Read the model definition and answer for the solid it produces. Units are mm, in the model's axes. Face numbers are marked on the shaded views. Give positions to 0.01 mm unless a question says otherwise; leave off trailing zeros. Write each loop counter-clockwise with the first axis right and the second up, starting at its lowest first coordinate (ties: lowest second). Pieces come first, ordered by that corner, then holes. Notation, with made-up numbers: (84.25, 69.5) - (88.25, 69.5) arc R13 ccw to (88.25, 83.5) - close; hole circle Ø9 at (-32, -11). An arc over 180 degrees is marked (long way). Answer as a JSON object with one key per item and string values. Group by question number.
```python
from build123d import *

# Parameters (mm, degrees)
F0_W     = 220
F0_H     = 50
F0_R     = 17.5
F0_R_2   = 7.5
F1_DEPTH = 20
F2_D     = 13.2
F3_R     = 5


with BuildPart() as f1:
    # F0 (on Top) → F1 (new body)
    with BuildSketch(Plane.XY):
        Rectangle(F0_W, F0_H)
        with Locations((-50, 0)):
            Circle(F0_R, mode=Mode.SUBTRACT)
        Circle(F0_R_2, mode=Mode.SUBTRACT)
        with Locations((50, 0)):
            Circle(F0_R, mode=Mode.SUBTRACT)
    extrude(amount=F1_DEPTH)

    # F2 (through all)
    with Locations(Plane(origin=(0, 0, 0), x_dir=(1, 0, 0), z_dir=(0, 0, -1))):
        with Locations((-95, -12.5), (-95, 12.5), (95, -12.5), (95, 12.5)):
            Hole(F2_D / 2)

    # F3
    f3_edges = [f1.edges().sort_by_distance(p)[0] for p in [
        (-110, -25, 10),
        (110, -25, 10),
        (110, 25, 10),
        (-110, 25, 10),
    ]]
    fillet(f3_edges, radius=F3_R)


solid = f1.part
```
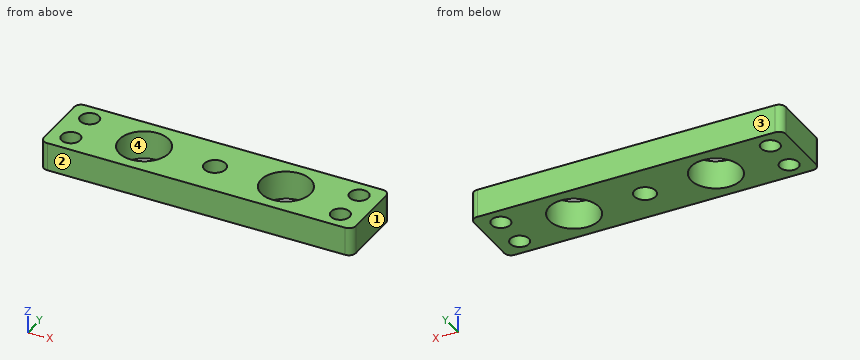
1) Find section D-D, the plane y = -12.5. Write down the section's boundary in (x, z), and give its area (3 significant figures).
2) Find section B-B, the plane y = 0. Write down the section's boundary in (x, z), and give its area (3 significant figures).
3) Find section C-C, the plane x = 0. Write down the section's boundary in (y, z), and give its area (3 significant figures).
4) Find the intervals of material crossed by line 1 (Y direction, x = -95, z = 12.25); line 2 (Y direction, x = -50, z = 8.25); line 3 (X direction, y = 2.5, z = 17.75), in increasing order. Write a range as [from, to].
5) For a pull along Y with two mould halves and no side action, classify the marked faces 1, 2, 3 and 4 as released by +Y, released by -Y, zero draft, split by the parting line, or undercut.
6) Find section A-A, the plane x = -95. Write down the section's boundary in (y, z).
Values follow:
{
 "1": {"outline": "(-110, 0) - (-101.6, 0) - (-101.6, 20) - (-110, 20) - close; (-88.4, 0) - (-62.25, 0) - (-62.25, 20) - (-88.4, 20) - close; (-37.75, 0) - (37.75, 0) - (37.75, 20) - (-37.75, 20) - close; (62.25, 0) - (88.4, 0) - (88.4, 20) - (62.25, 20) - close; (101.6, 0) - (110, 0) - (110, 20) - (101.6, 20) - close", "area": "2,890 mm2"},
 "2": {"outline": "(-110, 0) - (-67.5, 0) - (-67.5, 20) - (-110, 20) - close; (-32.5, 0) - (-7.5, 0) - (-7.5, 20) - (-32.5, 20) - close; (7.5, 0) - (32.5, 0) - (32.5, 20) - (7.5, 20) - close; (67.5, 0) - (110, 0) - (110, 20) - (67.5, 20) - close", "area": "2,700 mm2"},
 "3": {"outline": "(-25, 0) - (-7.5, 0) - (-7.5, 20) - (-25, 20) - close; (7.5, 0) - (25, 0) - (25, 20) - (7.5, 20) - close", "area": "700 mm2"},
 "4": {"line 1": "y = [-25, -19.1], [-5.9, 5.9], [19.1, 25]", "line 2": "y = [-25, -17.5], [17.5, 25]", "line 3": "x = [-110, -67.32], [-32.68, -7.07], [7.07, 32.68], [67.32, 110]"},
 "5": {"face 1": "zero draft", "face 2": "released by -Y", "face 3": "released by +Y", "face 4": "undercut"},
 "6": {"outline": "(-25, 0) - (-19.1, 0) - (-19.1, 20) - (-25, 20) - close; (-5.9, 0) - (5.9, 0) - (5.9, 20) - (-5.9, 20) - close; (19.1, 0) - (25, 0) - (25, 20) - (19.1, 20) - close"}
}
